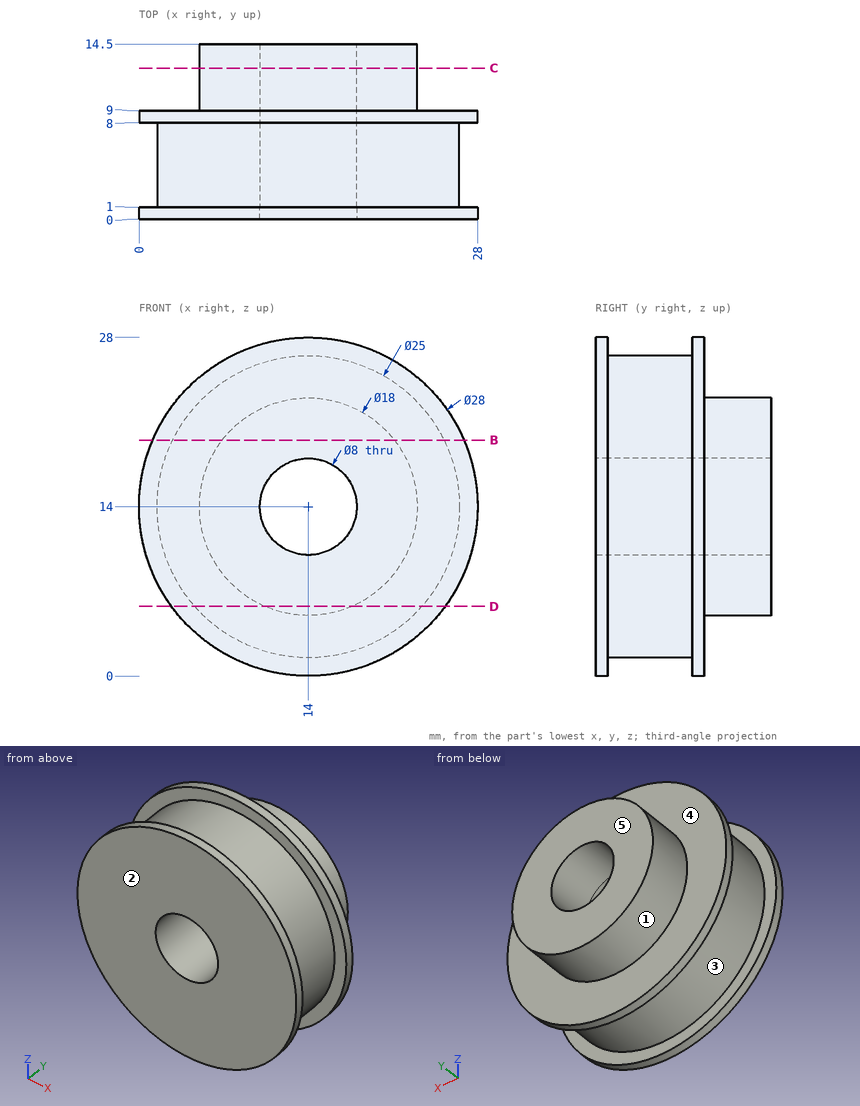
Can you work these out from the drawing? Everything is in mm from the part's minimum corner. A direction names the side the tool comes from. Coordinates: 2 decimals unless noted, no trailing zeros. Loops run counter-clockwise (first coordinate to the right, second up) from the corner with the lowest first, then second, coordinate; pieces in that order, holes last.
1. I need wall thicknesses on L1, parallel to Z at x = 14, y = 11.3; L2, parallel to X at y = 8.85, z = 14; L3, parallel to X at y = 2.5, z = 14. Which ranges of each line are inside material? Lowest first, please.
2. If we mould it in two halves opening along Y, with no side actions, what happens to the marked faces 1, 2 and 3? For each: pulls with the +Y half, pulls with the -Y half, needs draft (parallel to the pull), parting line crosses it, or undercut.
3. Imagine slicing it at C-C, the plane y = 12.5. Please give me the cut outline in (x, z).
4. Imagine slicing it at B-B, the plane z = 19.5. Please give me the cut outline in (x, y).
5. Imagine slicing it at D-D, the plane z = 5.75. Please give me the cut outline in (x, y).
6. For the marked faces 4 and 5, which set-ups out of +Z, -Z, +X, -X, +Y, -Y let a thin tool reach every point of the face, with its end or its side?
Taken from the geometry:
1. L1: z = 5 to 10, 18 to 23
1. L2: x = 0 to 10, 18 to 28
1. L3: x = 1.5 to 10, 18 to 26.5
2. face 1: needs draft
2. face 2: pulls with the -Y half
2. face 3: undercut
3. outline: circle Ø18 at (14, 14); hole circle Ø8 at (14, 14)
4. outline: (1.13, 0) - (26.87, 0) - (26.87, 1) - (25.22, 1) - (25.22, 8) - (26.87, 8) - (26.87, 9) - (21.12, 9) - (21.12, 14.5) - (6.88, 14.5) - (6.88, 9) - (1.13, 9) - (1.13, 8) - (2.78, 8) - (2.78, 1) - (1.13, 1) - close
5. outline: (2.69, 0) - (25.31, 0) - (25.31, 1) - (23.39, 1) - (23.39, 8) - (25.31, 8) - (25.31, 9) - (17.6, 9) - (17.6, 14.5) - (10.4, 14.5) - (10.4, 9) - (2.69, 9) - (2.69, 8) - (4.61, 8) - (4.61, 1) - (2.69, 1) - close
6. face 4: +Y
6. face 5: +Z, -Z, +X, -X, +Y
